Geometry: final body of the model. Coordinates: model frame, mm. Face numbers are marked on the shaded views. A direction names the side the tool comes from. Coordinates: 2 decimals unless noted, no trailing zeros. Order: outer loops, then holes, each group sorted by start corner. A loop starts at its lowest first (then second) coordinate and runs counter-clockwise, first axis right, second up. Notation, with made-up numbers: M -29.5,62 L -7.5,62 A27 cw -7.5,80 Z; hole C 82.25,25.25 d5. An arc over 180 degrees is marked long. Write item = value, one per line.
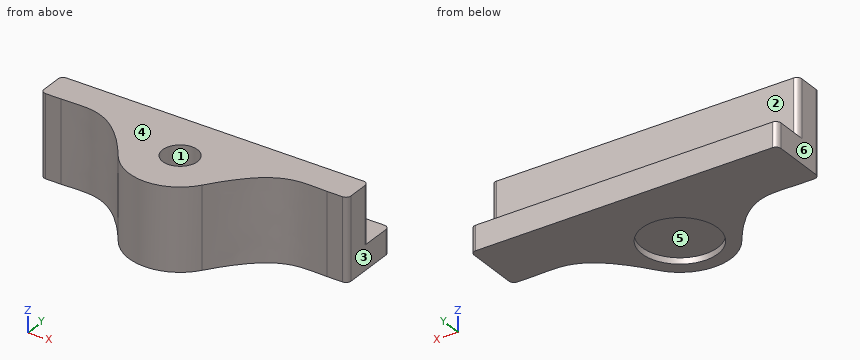
from build123d import *

# Parameters (mm, degrees)
SKETCH1_R           = 1.7
BOSS_EXTRUDE1_DEPTH = 8
SKETCH2_W           = 30
SKETCH2_H           = 3
CUT_EXTRUDE1_DEPTH  = 5.6
FILLET1_R           = 0.5
SKETCH5_R           = 3.7
CUT_EXTRUDE2_DEPTH  = 1
CHAMFER1_SIZE       = 2
SKETCH6_R           = 1.7
BOSS_EXTRUDE2_DEPTH = 0.4
BOSS_EXTRUDE3_START = -0.4
SKETCH7_R           = 3.7
BOSS_EXTRUDE3_DEPTH = 0.4


with BuildPart() as part:
    # Sketch1 → Boss-Extrude1 (new body)
    with BuildSketch(Plane.XY):
        with BuildLine():
            Line((20, 6), (20, 0))
            Line((20, 0), (18, 0))
            add(Edge.make_bspline(
                [(18, 0), (15.260318753, 0), (13.131354564, 0.908049894), (9.098678762, -4.863709553)],
                knots=[0, 0, 0, 0, 1, 1, 1, 1], degree=3))
            ThreePointArc((9.098678762, -4.863709553), (5, -7), (0.901321238, -4.863709553))
            add(Edge.make_bspline(
                [(-8, 0), (-5.260318753, 0), (-3.131354564, 0.908049894), (0.901321238, -4.863709553)],
                knots=[0, 0, 0, 0, 1, 1, 1, 1], degree=3))
            Line((-8, 0), (-10, 0))
            Line((-10, 0), (-10, 6))
            Line((-10, 6), (20, 6))
        make_face()
        with Locations((5, -2)):
            Circle(SKETCH1_R, mode=Mode.SUBTRACT)
    extrude(amount=BOSS_EXTRUDE1_DEPTH)

    # Sketch2 → Cut-Extrude1 (cut)
    with BuildSketch(Plane.XY.offset(8)):
        with Locations((5, 4.5)):
            Rectangle(SKETCH2_W, SKETCH2_H)
    extrude(amount=-CUT_EXTRUDE1_DEPTH, mode=Mode.SUBTRACT)

    # Fillet1
    fillet1_edges = [part.edges().sort_by_distance(p)[0] for p in [
        (20, 0, 4),
        (-10, 0, 4),
        (20, 6, 1.2),
        (-10, 6, 1.2),
        (20, 3, 5.2),
        (-10, 3, 5.2),
    ]]
    fillet(fillet1_edges, radius=FILLET1_R)

    # Sketch5 → Cut-Extrude2 (cut)
    with BuildSketch(Plane(origin=(0, 0, 0), x_dir=(-1, 0, 0), z_dir=(0, 0, -1))):
        with Locations((-5, -2)):
            Circle(SKETCH5_R)
    extrude(amount=-CUT_EXTRUDE2_DEPTH, mode=Mode.SUBTRACT)

    # Chamfer1
    chamfer1_edges = [part.edges().sort_by_distance(p)[0] for p in [
        (3.3, -2, 1),
    ]]
    chamfer(chamfer1_edges, length=CHAMFER1_SIZE - 0.0001)  # a hair under: the kernel refuses the full size

    # Sketch6 → Boss-Extrude2 (add)
    with BuildSketch(Plane.XY.offset(3)):
        with Locations((5, -2)):
            Circle(SKETCH6_R)
    extrude(amount=BOSS_EXTRUDE2_DEPTH)

    # Sketch7 → Boss-Extrude3 (add)
    with BuildSketch(Plane.XY.offset(1).offset(BOSS_EXTRUDE3_START)):
        with Locations(Location((5, -2, 0), (0, 0, 180))):
            Circle(SKETCH7_R)
    extrude(amount=BOSS_EXTRUDE3_DEPTH)


solid = part.part
1) Set-up query: the marked faces 1, 2 and 3. Return all of +Z, -Z, +X, -X, +Y, -Y with unobstructed straight access to the full face (end or side cutting, diameter ignored); none if empty.
Numbers:
face_1 = +Z
face_2 = +Z, +X, -X, +Y
face_3 = +Z, -Z, +X, +Y, -Y
2) Pin query (flat end, axial travel): pin 1 (2.5 mm diameter, centred on x = 5, y = -2, fed in from +Z); pin 2 (1.6 mm diameter, centred on x = -9, z = 5, fed in from -Y); pin 3 (1 mm diameter, centred on x = 8, z = 6, fed in from -Y). Return the tip coordinate at first contact, or that it passes through.
Numbers:
pin_1 = 3.4
pin_2 = 0
pin_3 = -6.33
3) Mould query, pull axis X, two halves, no side actions, for the marked faces 4, 5 and 6. Classes: pulls with the +X half, pulls with the -X half, needs draft (parallel to the pull), parting line crosses it, or undercut.
Numbers:
face_4 = needs draft
face_5 = undercut
face_6 = pulls with the -X half
4) Line query: L1, parallel to Y at x = 5, z = 5.1; L2, parallel to Y at x = 5, z = 0.35; L3, parallel to Y at x = 5, z = 3.05. Output: solid intervals per line, ascending.
Numbers:
L1 = -7 to -3.7, -0.3 to 3
L2 = -7 to -5.7, 1.7 to 6
L3 = -7 to 3
5) Section B-B, the plane y = 4. Return loops of the section in (x, z), and give its area (3 significant figures).
Numbers:
outline = M -10,0 L 20,0 L 20,2.4 L -10,2.4 Z
area = 72.0 mm²
